Job drawing, mm, ordinate dimensions from the low corner. One solid piece. Coordinates: 2 decimals unless noted, no trailing zeros. Write each loop counter-clockwise with the first axis right and the second up, starting at its lowest first coordinate (ties: lowest second). Pieces come first, ordered by that corner, then holes.
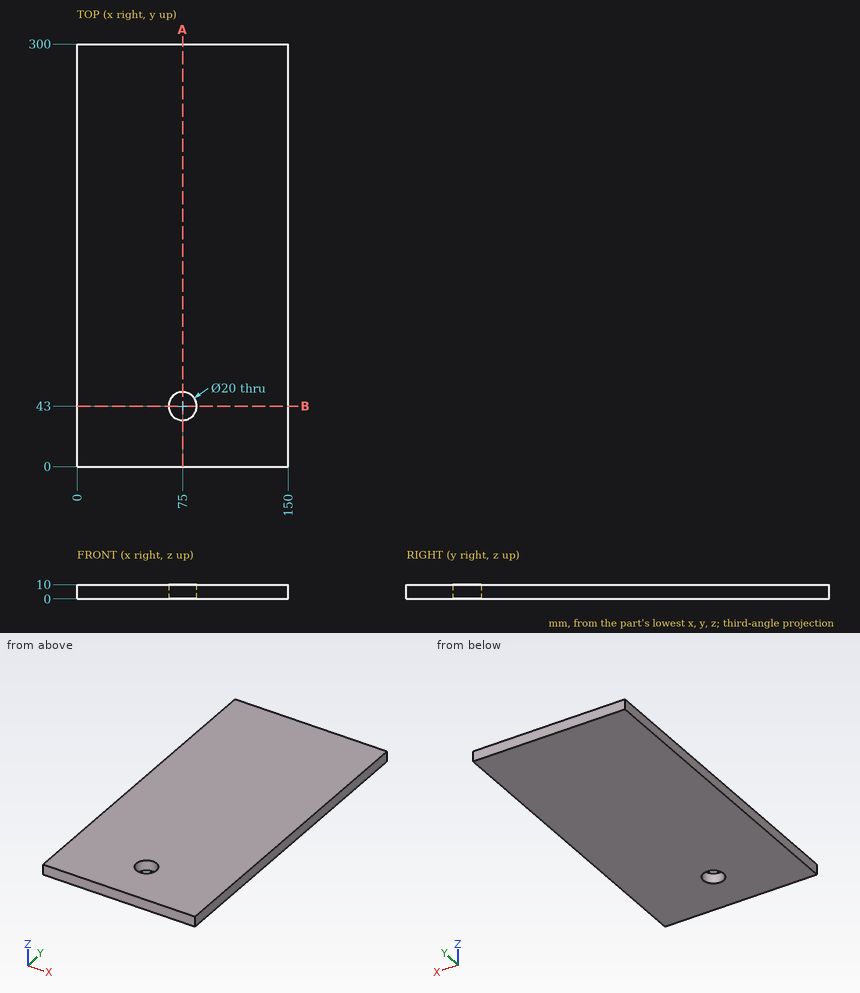
1. Saw through at A-A on x = 75. List the corners of the cut face in (y, z), plus the area to 3 significant figures.
Computed values:
outline: (0, 0) - (33, 0) - (33, 10) - (0, 10) - close; (53, 0) - (300, 0) - (300, 10) - (53, 10) - close
area: 2,800 mm2
2. Probe line 1 along Y through (x, z) = (75, 5.25); line 2 along X through (y, z) = (39, 4.5). List the from-to ranges inside material, lowest first.
Computed values:
line 1: y = 0 to 33, 53 to 300
line 2: x = 0 to 65.83, 84.17 to 150
3. Saw through at B-B on y = 43. List the corners of the cut face in (x, z), plus the area to 3 significant figures.
Computed values:
outline: (0, 0) - (65, 0) - (65, 10) - (0, 10) - close; (85, 0) - (150, 0) - (150, 10) - (85, 10) - close
area: 1,300 mm2
